from build123d import *

# Parameters (mm, degrees)
BOSS_EXTRUDE1_DEPTH = 0.7
BOSS_EXTRUDE2_DEPTH = 0.3
FILLET1_R           = 0.7
CHAMFER1_SIZE2      = 0.3
CHAMFER1_SIZE       = 0.173205081
SKETCH3_W           = 0.8
SKETCH3_H           = 3
BOSS_EXTRUDE3_DEPTH = 0.01
LPATTERN1_COUNT     = 8
LPATTERN1_PITCH     = 1
CUT_EXTRUDE1_START  = -0.01
CUT_EXTRUDE1_DEPTH  = 0.01
BOSS_EXTRUDE4_DEPTH = 0.01


with BuildPart() as part:
    # Sketch1 → Boss-Extrude1 (new body)
    with BuildSketch(Plane(origin=(0, 0, 0), x_dir=(1, 0, 0), z_dir=(0, 1, 0))):
        Polygon((6, -2.5), (6, -7.5), (-5, -7.5), (-5, 7.5), (4.5, 7.5), (4.5, 2.5), (6, 1), (6, -0.5), (5.3, -0.5), (5.3, -1.5), align=None)
    extrude(amount=BOSS_EXTRUDE1_DEPTH)

    # Sketch2 → Boss-Extrude2 (add)
    with BuildSketch(Plane(origin=(0, 0.7, 0), x_dir=(1, 0, 0), z_dir=(0, 1, 0))):
        with BuildLine():
            Line((-5, -6.3), (-5, -7.5))
            Line((-5, -7.5), (6, -7.5))
            Line((6, -7.5), (6, -6.3))
            ThreePointArc((6, -6.3), (0.5, -5.6), (-5, -6.3))
        make_face()
    extrude(amount=BOSS_EXTRUDE2_DEPTH)

    # Fillet1
    fillet1_edges = [part.edges().sort_by_distance(p)[0] for p in [
        (6, 0.5, 7.5),
        (-5, 0.5, 7.5),
        (-5, 0.35, -7.5),
        (4.5, 0.35, -7.5),
    ]]
    fillet(fillet1_edges, radius=FILLET1_R)

    # Chamfer1
    chamfer1_edges = [part.edges().sort_by_distance(p)[0] for p in [
        (0.5, 1, 5.6),
    ]]
    chamfer1_side = [part.faces().sort_by_distance(p)[0] for p in [
        (0.5, 1, 5.603464102),
    ]]
    chamfer(chamfer1_edges, length=CHAMFER1_SIZE - 0.0001, length2=CHAMFER1_SIZE2 - 0.0001, reference=chamfer1_side[0])  # a hair under: the kernel refuses the full size

    # Sketch3 → Boss-Extrude3 (add)
    with BuildSketch(Plane.XZ):
        with Locations((-3.8, -5)):
            Rectangle(SKETCH3_W, SKETCH3_H)
    boss_extrude3 = extrude(amount=BOSS_EXTRUDE3_DEPTH)

    # LPattern1: Boss-Extrude3 ×8
    with Locations(*[(i * LPATTERN1_PITCH, 0, 0) for i in range(1, LPATTERN1_COUNT)]):
        add(boss_extrude3)

    # Sketch5 → Cut-Extrude1 (cut)
    with BuildSketch(Plane(origin=(0, 0.7, 0), x_dir=(1, 0, 0), z_dir=(0, 1, 0)).offset(CUT_EXTRUDE1_START)):
        with BuildLine():
            Line((-5, -6.3), (-5, 7.687555769))
            Line((-5, 7.687555769), (-2, 7.687555769))
            Line((-2, 7.687555769), (-2, -5.742786977))
            ThreePointArc((-2, -5.742786977), (-3.509690959, -5.969217972), (-5, -6.3))
        make_face()
    extrude(amount=CUT_EXTRUDE1_DEPTH, mode=Mode.SUBTRACT)

    # Sketch4 → Boss-Extrude4 (add)
    # profile 1 of 2: a face of its own
    with BuildSketch(Plane(origin=(0, 0.7, 0), x_dir=(1, 0, 0), z_dir=(0, 1, 0))):
        with BuildLine():
            Line((-0.615384615, -2.75), (-0.37109375, -2.439002404))
            Line((-0.37109375, -2.439002404), (1.447115385, -3.628004808))
            add(Edge.make_bspline(
                [(1.447115385, -3.628004808), (1.434497564, -3.548843023), (1.409885078, -3.394429011), (1.405824862, -3.238129999), (1.403846154, -3.161959135)],
                knots=[0, 0, 0, 0, 1.025318673, 2, 2, 2, 2], degree=3))
            add(Edge.make_bspline(
                [(1.403846154, -3.161959135), (1.40507544, -3.116223068), (1.407495254, -3.026192981), (1.426117348, -2.894012808), (1.455463919, -2.766998457), (1.498242541, -2.645676402), (1.552888396, -2.529611073), (1.618381342, -2.418136818), (1.698102499, -2.313347546), (1.787159106, -2.21389978), (1.885789037, -2.12359384), (1.990470293, -2.043703676), (2.101194596, -1.97622976), (2.217937047, -1.922472915), (2.339783801, -1.879511677), (2.46721007, -1.848928505), (2.600430921, -1.830645424), (2.691048417, -1.828176974), (2.737079327, -1.826923077)],
                knots=[0, 0, 0, 0, 1.043709831, 2.054511743, 3.041122595, 4.01515914, 4.98481438, 5.965901842, 6.960491961, 7.985277438, 9.0096037, 10.00832444, 10.987059228, 11.962929573, 12.936966118, 13.931840027, 14.949438142, 16, 16, 16, 16], degree=3))
            add(Edge.make_bspline(
                [(2.737079327, -1.826923077), (2.800055589, -1.828748336), (2.923977968, -1.832340015), (3.104428638, -1.868279847), (3.276237792, -1.923709962), (3.436432503, -2.004206562), (3.586122296, -2.102297304), (3.718320331, -2.223387248), (3.836219906, -2.361468581), (3.934767808, -2.517682681), (4.015260324, -2.685776222), (4.073072014, -2.862372856), (4.108665247, -3.045750298), (4.113127423, -3.170213408), (4.115384615, -3.233173077)],
                knots=[0, 0, 0, 0, 1.031403119, 2.029557249, 3.004870281, 3.983165322, 4.960181699, 5.929903783, 6.912123683, 7.928973898, 8.949315281, 9.960468141, 10.968302741, 12, 12, 12, 12], degree=3))
            add(Edge.make_bspline(
                [(4.115384615, -3.233173077), (4.113425363, -3.293728526), (4.109544427, -3.413678269), (4.074792271, -3.590083158), (4.018865585, -3.759886916), (3.940200981, -3.920909877), (3.842516001, -4.070320901), (3.725735923, -4.205059604), (3.589698509, -4.321514883), (3.437379658, -4.419302266), (3.273930698, -4.497189895), (3.103206109, -4.555053217), (2.925922629, -4.589030783), (2.805730368, -4.59376788), (2.745192308, -4.596153846)],
                knots=[0, 0, 0, 0, 1.012172929, 2.004937354, 2.995255351, 3.995689452, 4.993936421, 5.973737378, 6.968231049, 7.979117505, 8.993136101, 9.989812463, 10.987515067, 12, 12, 12, 12], degree=3))
            add(Edge.make_bspline(
                [(2.745192308, -4.596153846), (2.698849272, -4.594634845), (2.604225648, -4.591533336), (2.460914755, -4.569877549), (2.31427765, -4.535079955), (2.189879401, -4.496109639), (2.08797173, -4.454933854), (2.005810099, -4.420666303), (1.921260148, -4.378014023), (1.831422616, -4.332533961), (1.738612774, -4.280132273), (1.641279485, -4.223155009), (1.54097072, -4.160026886), (1.472899612, -4.115772392), (1.438100962, -4.093149038)],
                knots=[0, 0, 0, 0, 1.173818275, 2.396712641, 3.66331629, 4.989737886, 5.693666774, 6.447286557, 7.243889047, 8.091586357, 8.998013824, 9.943181721, 10.948533338, 12, 12, 12, 12], degree=3))
            Line((1.438100962, -4.093149038), (-0.615384615, -2.75))
        make_face()
        with BuildLine():
            add(Edge.make_bspline(
                [(1.865384615, -3.246694712), (1.8663753, -3.28097808), (1.868310394, -3.347943459), (1.879792233, -3.446134849), (1.900690488, -3.539368105), (1.929667741, -3.627670289), (1.965393302, -3.711586134), (2.011232334, -3.789452661), (2.064624344, -3.862872186), (2.125472743, -3.930671657), (2.192048636, -3.992157699), (2.263368863, -4.045103926), (2.337700822, -4.090775827), (2.415669188, -4.12790953), (2.497243218, -4.156825359), (2.582047978, -4.177741676), (2.670652083, -4.189382215), (2.73073673, -4.191318798), (2.761418269, -4.192307692)],
                knots=[0, 0, 0, 0, 1.129656352, 2.206547016, 3.251334079, 4.271920891, 5.265058649, 6.249872215, 7.241923875, 8.251504132, 9.246416584, 10.222533834, 11.173322129, 12.116503788, 13.062124155, 14.020151864, 14.989013135, 16, 16, 16, 16], degree=3))
            add(Edge.make_bspline(
                [(2.761418269, -4.192307692), (2.791820074, -4.191473852), (2.851730559, -4.189830668), (2.939673033, -4.175840608), (3.024108675, -4.153478957), (3.10472016, -4.121176044), (3.183055016, -4.08192157), (3.256667917, -4.031535431), (3.327943341, -3.973706783), (3.393569596, -3.906186554), (3.454494335, -3.833170458), (3.50796717, -3.755324944), (3.553183997, -3.673822107), (3.590651134, -3.588896682), (3.618232291, -3.499498881), (3.639347167, -3.4070803), (3.650890957, -3.3103844), (3.652848159, -3.244919557), (3.653846154, -3.211538462)],
                knots=[0, 0, 0, 0, 0.989367052, 1.949669134, 2.891858276, 3.827522767, 4.772653562, 5.738670152, 6.725809442, 7.756636004, 8.798867547, 9.819240912, 10.826537776, 11.829883227, 12.835515726, 13.868058748, 14.912904531, 16, 16, 16, 16], degree=3))
            add(Edge.make_bspline(
                [(3.653846154, -3.211538462), (3.652848082, -3.178157421), (3.650890727, -3.112692685), (3.639348041, -3.015996006), (3.618229086, -2.9235803), (3.590662748, -2.834172058), (3.553140653, -2.749285358), (3.508250138, -2.667853764), (3.454166469, -2.590744499), (3.393674202, -2.517680886), (3.32756834, -2.45044126), (3.257310144, -2.391252543), (3.182466, -2.342440577), (3.105028171, -2.301629691), (3.024060526, -2.269684452), (2.939686174, -2.247212711), (2.85172713, -2.233252413), (2.79181892, -2.231605144), (2.761418269, -2.230769231)],
                knots=[0, 0, 0, 0, 1.087281468, 2.132306021, 3.165025708, 4.170830268, 5.174347389, 6.181816599, 7.194310624, 8.23672049, 9.267723423, 10.261267456, 11.222032883, 12.171822355, 13.107646935, 14.049997283, 15.01046367, 16, 16, 16, 16], degree=3))
            add(Edge.make_bspline(
                [(2.761418269, -2.230769231), (2.730696704, -2.23147675), (2.670400261, -2.232865381), (2.582087612, -2.248571602), (2.496812336, -2.270354649), (2.415110442, -2.303247134), (2.337304096, -2.345979773), (2.263001203, -2.398030102), (2.191628428, -2.458242489), (2.125342463, -2.527800045), (2.064690312, -2.603502471), (2.011305764, -2.684058006), (1.965736495, -2.767997769), (1.929778734, -2.856504174), (1.900810753, -2.948386374), (1.879866743, -3.044278828), (1.868340324, -3.144249739), (1.866382401, -3.212111437), (1.865384615, -3.246694712)],
                knots=[0, 0, 0, 0, 0.978259475, 1.920005202, 2.851759169, 3.7803069, 4.719124913, 5.675758531, 6.668034766, 7.691045932, 8.733780038, 9.756656648, 10.768121246, 11.773215211, 12.79725739, 13.836288844, 14.897342417, 16, 16, 16, 16], degree=3))
        make_face(mode=Mode.SUBTRACT)
    # profile 2 of 2: a face of its own
    with BuildSketch(Plane(origin=(0, 0.7, 0), x_dir=(1, 0, 0), z_dir=(0, 1, 0))):
        Polygon((-0.615384615, 1.091045673), (-0.615384615, 1.173076923), (2.5, 1.173076923), (2.5, 1.692307692), (2.961538462, 1.692307692), (2.961538462, 1.173076923), (4, 1.173076923), (4, 0.769230769), (2.961538462, 0.769230769), (2.961538462, -1.365384615), align=None)
        Polygon((2.5, 0.769230769), (0.545673077, 0.769230769), (2.5, -0.572115385), align=None, mode=Mode.SUBTRACT)
    extrude(amount=BOSS_EXTRUDE4_DEPTH)


solid = part.part
Work out the finished part from the listing and answer in its coordinate system (mm). A direction names the side the tool comes from. Give positions to 0.01 mm unless a question says otherwise; leave off trailing zeros. Write each loop counter-clockwise with the first axis right and the second up, starting at its lowest first coordinate (ties: lowest second). Pieces come first, ordered by that corner, then holes.
Q1. A tool of negligible diameter and unlimited length cuts with its end or side. For faces 1 (the face through (0.4, 0.5, 7.5)), 2 (the face through (-3, 0.69, -1)), from which of +Z, -Z, +X, -X, +Y, -Y can it reach the whole face along a straight path? Write none if from no direction.
Answer:
face 1: +Z, +X, -X, +Y, -Y
face 2: -Z, -X, +Y
Q2. Straight lines are drawn through the part: L1, parallel to Y at x = 1, z = 4; L2, parallel to Y at x = -4, z = 6.5; L3, parallel to X at y = 0.15, z = -4.5. For each, find the intervals that lie inside material, in ascending order.
Answer:
L1: y = 0 to 0.7
L2: y = 0 to 1
L3: x = -5 to 4.5
Q3. The part is cut by section A-A on y = 0.2. Give the vertices of the cut face in (x, z), and give its area (3 significant figures).
Answer:
outline: (-5, -6.8) arc R0.7 ccw to (-4.3, -7.5) - (3.8, -7.5) arc R0.7 ccw to (4.5, -6.8) - (4.5, -2.5) - (6, -1) - (6, 0.5) - (5.3, 0.5) - (5.3, 1.5) - (6, 2.5) - (6, 6.8) arc R0.7 ccw to (5.3, 7.5) - (-4.3, 7.5) arc R0.7 ccw to (-5, 6.8) - close
area: 155 mm2
Q4. Given pin 1 (1.5 mm diameter, centred on x = -2.5, z = 2.5, fed in from -Y), flat-ended and moving along its own axis, determine where the tip first touches the part or whether it passes through.
Answer:
pin 1: stops at y = 0
